CAD build for the part. Positions are in the model's coordinates, mm. Give positions to 0.01 mm unless a question says otherwise; leave off trailing zeros. Order: outer loops, then holes, each group sorted by start corner. A loop starts at its lowest first (then second) coordinate and runs counter-clockwise, first axis right, second up.
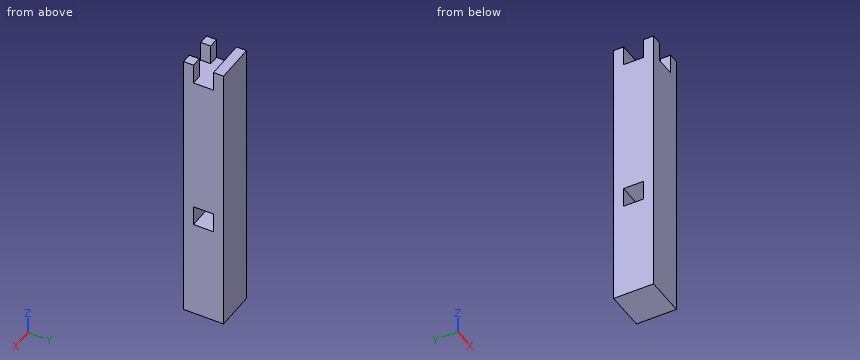
from build123d import *

# Parameters (mm, degrees)
F0_W     = 101.6
F0_H     = 711.2
F1_DEPTH = 101.6
F3_W     = 50.8
F3_H     = 50.8
F4_DEPTH = 101.6
F2_W     = 50.8
F2_H     = 50.8
F5_DEPTH = 25.4
F7_DEPTH = 101.6


with BuildPart() as f1:
    # F0 (on Front) → F1 (new body)
    with BuildSketch(Plane.XZ):
        Rectangle(F0_W, F0_H)
    extrude(amount=F1_DEPTH)

    # F3 (on face) → F4 (cut)
    with BuildSketch(Plane.YZ.offset(50.8)):
        with Locations((-50.8, 330.2)):
            Rectangle(F3_W, F3_H)
    extrude(amount=-F4_DEPTH, mode=Mode.SUBTRACT)

    # F2 (on face) → F5 (cut)
    with BuildSketch(Plane.XZ.offset(101.6)):
        with Locations((0, 330.2)):
            Rectangle(F2_W, F2_H)
    extrude(amount=-F5_DEPTH, mode=Mode.SUBTRACT)

    # F6 (on face) → F7 (cut)
    with BuildSketch(Plane(origin=(-50.8, 0, 0), x_dir=(0, -1, 0), z_dir=(-1, 0, 0))):
        Polygon((50.8, -101.6), (76.2, -101.6), (76.2, -50.8), (25.4, -50.8), (25.4, -101.6), align=None)
    extrude(amount=-F7_DEPTH, mode=Mode.SUBTRACT)


solid = f1.part
1. Pin check, flat tips, straight feed: P1, Ø12.5, axis at x = 39, z = 337, coming from the +Y side; P2, Ø4, axis at x = 40, y = -34.5, coming from the +Z side. Stop position of each tip, or through.
2. Wall check: line 1 (Z direction, x = 34.5, y = -75); line 2 (Z direction, x = -4, y = -80). Give the ranges that are in metal, low to high.
3. Saw through at D-D on x = 5.5. Give the cut face in (y, z).
4. Saw through at C-C on y = -83. Give the cut face in (x, z).
5. Saw through at B-B on y = -49.5. Give the cut face in (x, z), plus the area to 3 significant figures.
6. Saw through at A-A on x = 33. Give the cut face in (y, z).
Reported:
1. P1: stops at y = 0
1. P2: stops at z = 304.8
2. line 1: z = -355.6 to -101.6, -50.8 to 304.8
2. line 2: z = -355.6 to 304.8
3. outline: (-101.6, -355.6) - (0, -355.6) - (0, 355.6) - (-25.4, 355.6) - (-25.4, 304.8) - (-101.6, 304.8) - close; hole (-76.2, -101.6) - (-25.4, -101.6) - (-25.4, -50.8) - (-76.2, -50.8) - close
4. outline: (-50.8, -355.6) - (50.8, -355.6) - (50.8, 355.6) - (25.4, 355.6) - (25.4, 304.8) - (-25.4, 304.8) - (-25.4, 355.6) - (-50.8, 355.6) - close
5. outline: (-50.8, -355.6) - (50.8, -355.6) - (50.8, -101.6) - (-50.8, -101.6) - close; (-50.8, -50.8) - (50.8, -50.8) - (50.8, 304.8) - (-50.8, 304.8) - close
5. area: 61,900 mm2
6. outline: (-101.6, -355.6) - (0, -355.6) - (0, 355.6) - (-25.4, 355.6) - (-25.4, 304.8) - (-76.2, 304.8) - (-76.2, 355.6) - (-101.6, 355.6) - close; hole (-76.2, -101.6) - (-25.4, -101.6) - (-25.4, -50.8) - (-76.2, -50.8) - close
